Can you work these out from the model? Positions are in its coordinate system, mm. Face numbers are marked on the shaded views. A direction names the side the tool comes from. Round coordinates to 2 decimals unless told otherwise and drop trailing zeros. Write each loop counter-clockwise with the first axis right and the second up, starting at its lowest first coordinate (ties: lowest second). Pieces come first, ordered by that corner, then holes.
Q1. If we section it at D-D (y = 40): Please give me the cut outline in (x, z).
Q2. If we section it at A-A (x = -25): Please give me the cut outline in (y, z).
Q3. For the marked faces 5 and 6, which set-ups out of +Z, -Z, +X, -X, +Y, -Y let a thin tool reach every point of the face, with its end or its side?
Q4. I'm going to push flat-ended pins straight in: pin 1 Ø3.5 at (y, z) = (39, -2) entering from -X; pin 2 Ø17 at (x, y) = (-25, 15) entering from -Z. Where does each tip first touch, or does it pass through?
Q5. If we section it at B-B (y = 15): Please give me the cut outline in (x, z).
Q6. If we section it at C-C (z = -2.5): Please give me the cut outline in (x, y), plus the area to 3 significant figures.
Q7. Please list where these lines run through material, in increasing order: line 1 along Z through (x, y) = (-30.25, 40); line 2 along Y through (x, z) = (-21.5, -6); line 3 along Y through (x, z) = (-21.75, 3).
Q8. We'd pull the mould along Y, two halves only. Please class the marked faces 1, 2, 3 and 4: +Y half, -Y half, draft (parallel to the pull), parting line (faces both ways), or undercut.
from build123d import *

# Parameters (mm, degrees)
SKETCH1_W           = 50
SKETCH1_H           = 70
BOSS_EXTRUDE1_DEPTH = 10
SKETCH2_R           = 7.5
CUT_EXTRUDE1_DEPTH  = 10
SKETCH3_W           = 50
SKETCH3_H           = 70
BOSS_EXTRUDE2_DEPTH = 40
SKETCH4_R           = 10.5
CUT_EXTRUDE3_DEPTH  = 40
SKETCH5_W           = 10
SKETCH5_H           = 70
CUT_EXTRUDE4_DEPTH  = 50
SKETCH6_R           = 6
CUT_EXTRUDE5_DEPTH  = 20
SKETCH7_W           = 50
SKETCH7_H           = 15
CUT_EXTRUDE6_DEPTH  = 30


with BuildPart() as part:
    # Sketch1 → Boss-Extrude1 (new body)
    with BuildSketch(Plane.XY):
        with Locations((-25, 35)):
            Rectangle(SKETCH1_W, SKETCH1_H)
    extrude(amount=BOSS_EXTRUDE1_DEPTH)

    # Sketch2 → Cut-Extrude1 (cut)
    with BuildSketch(Plane.XY.offset(10)):
        with Locations((-25, 15)):
            Circle(SKETCH2_R)
    extrude(amount=-CUT_EXTRUDE1_DEPTH, mode=Mode.SUBTRACT)

    # Sketch3 → Boss-Extrude2 (add)
    with BuildSketch(Plane(origin=(0, 0, 0), x_dir=(-1, 0, 0), z_dir=(0, 0, -1))):
        with Locations((25, 35)):
            Rectangle(SKETCH3_W, SKETCH3_H)
    extrude(amount=BOSS_EXTRUDE2_DEPTH)

    # Sketch4 → Cut-Extrude3 (cut)
    with BuildSketch(Plane(origin=(0, 0, -40), x_dir=(-1, 0, 0), z_dir=(0, 0, -1))):
        with Locations((25, 15)):
            Circle(SKETCH4_R)
    extrude(amount=-CUT_EXTRUDE3_DEPTH, mode=Mode.SUBTRACT)

    # Sketch5 → Cut-Extrude4 (cut)
    with BuildSketch(Plane(origin=(0, 0, -40), x_dir=(-1, 0, 0), z_dir=(0, 0, -1))):
        with Locations((5, 35)):
            Rectangle(SKETCH5_W, SKETCH5_H)
        with Locations((45, 35)):
            Rectangle(SKETCH5_W, SKETCH5_H)
    extrude(amount=-CUT_EXTRUDE4_DEPTH, mode=Mode.SUBTRACT)

    # Sketch6 → Cut-Extrude5 (cut)
    with BuildSketch(Plane.ZY.offset(40)):
        with Locations(Location((-27.5, 40, 0), (0, 0, 270))):
            Circle(SKETCH6_R)
        with Locations(Location((-2.5, 40, 0), (0, 0, 270))):
            Circle(SKETCH6_R)
    extrude(amount=-CUT_EXTRUDE5_DEPTH, mode=Mode.SUBTRACT)

    # Sketch7 → Cut-Extrude6 (cut)
    with BuildSketch(Plane.ZY.offset(40)):
        with Locations((-15, 62.5)):
            Rectangle(SKETCH7_W, SKETCH7_H)
    extrude(amount=-CUT_EXTRUDE6_DEPTH, mode=Mode.SUBTRACT)


solid = part.part
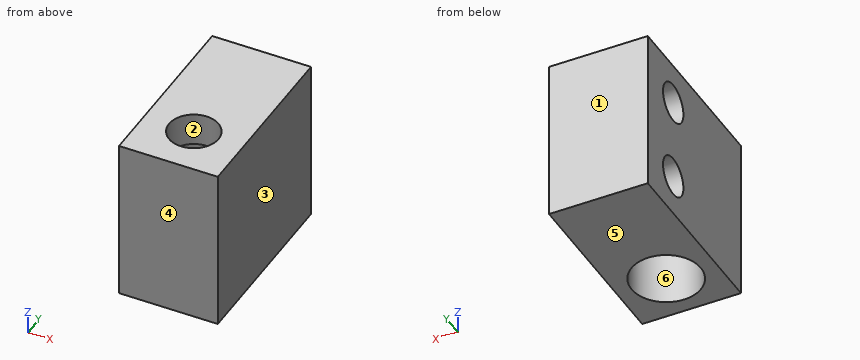
A:
1. outline: (-40, -40) - (-10, -40) - (-10, 10) - (-40, 10) - (-40, 3.5) - (-20, 3.5) - (-20, -8.5) - (-40, -8.5) - (-40, -21.5) - (-20, -21.5) - (-20, -33.5) - (-40, -33.5) - close
2. outline: (0, -40) - (4.5, -40) - (4.5, 0) - (7.5, 0) - (7.5, 10) - (0, 10) - close; (22.5, 0) - (25.5, 0) - (25.5, -40) - (55, -40) - (55, 10) - (22.5, 10) - close; hole circle Ø12 at (40, -27.5); hole circle Ø12 at (40, -2.5)
3. face 5: -Z, +X, -X, +Y, -Y
3. face 6: -Z
4. pin 1: stops at x = -20
4. pin 2: stops at z = 0
5. outline: (-40, -40) - (-35.5, -40) - (-35.5, 0) - (-32.5, 0) - (-32.5, 10) - (-40, 10) - close; (-17.5, 0) - (-14.5, 0) - (-14.5, -40) - (-10, -40) - (-10, 10) - (-17.5, 10) - close
6. outline: (-40, 0) - (-10, 0) - (-10, 55) - (-40, 55) - (-40, 46) - (-20, 46) - (-20, 34) - (-40, 34) - close; hole circle Ø21 at (-25, 15)
6. area: 1,060 mm2
7. line 1: z = -40 to -33.5, -21.5 to -8.5, 3.5 to 10
7. line 2: y = 0 to 5.1, 24.9 to 35.13, 44.87 to 55
7. line 3: y = 0 to 8.24, 21.76 to 37.6, 42.4 to 55
8. face 1: +Y half
8. face 2: undercut
8. face 3: draft
8. face 4: -Y half
